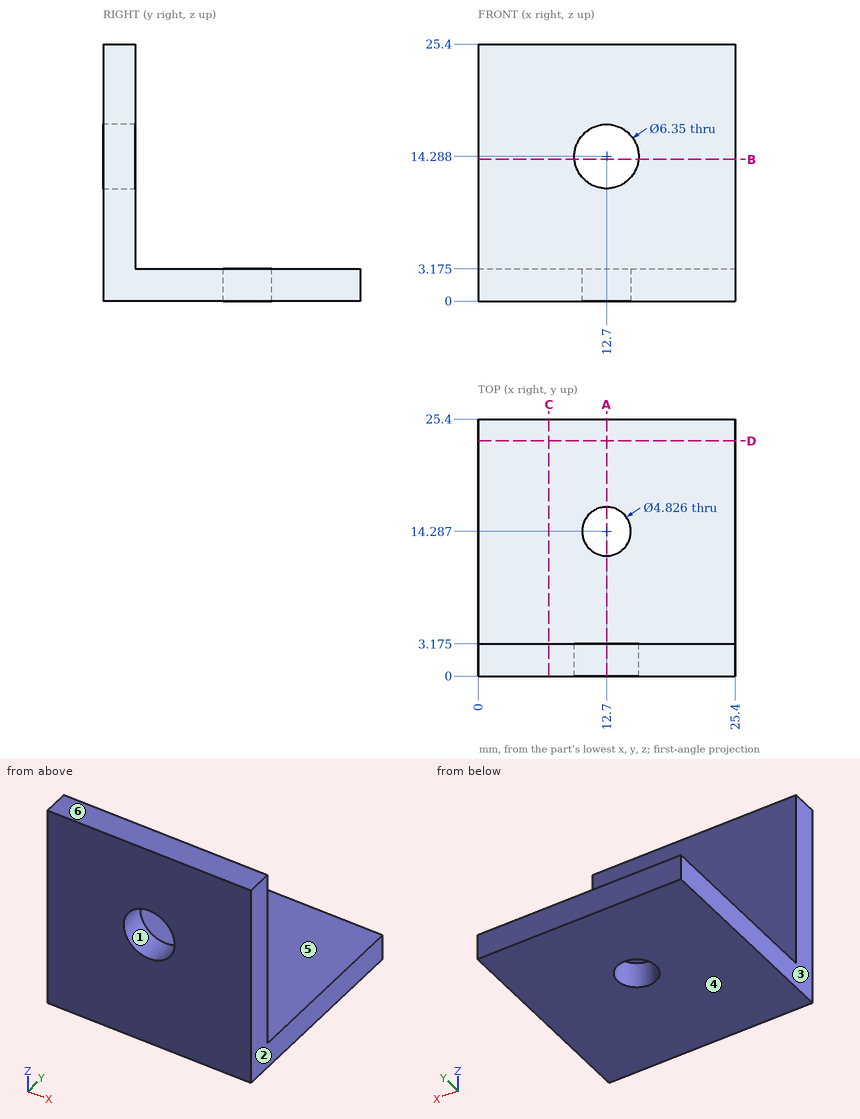
Part print with two shaded views. Sizes in mm from the minimum x, y, z corner. A direction names the side the tool comes from. Round coordinates to 2 decimals unless told otherwise and drop trailing zeros. Write each loop counter-clockwise with the first axis right and the second up, starting at its lowest first coordinate (ties: lowest second). Pieces come first, ordered by that corner, then holes. Notation, with made-up numbers: M 87.25,65.25 L 143.25,65.25 A19 ccw 143.25,72.25 Z; hole C 76.5,15.25 d10. An arc over 180 degrees is marked long. Put each result on its own line as item: value. Start each with the question number.
1) Saw through at B-B, the plane z = 14. Write the cut outline in (x, y) (1 decimal).
2) Saw through at C-C, the plane x = 7. Write the cut outline in (y, z) (1 decimal).
3) Drill centre lines: probe 1 along Y at (x, z) = (12.7, 1.45) (1 decimal); probe 2 along Z at (x, y) = (12, 18.5) (1 decimal). Where is each one in solid material? Low to high. Write a range as [from, to].
4) Saw through at A-A, the plane x = 12.7. Write the cut outline in (y, z) (1 decimal).
5) Saw through at D-D, the plane y = 23.25. Write the cut outline in (x, z) (1 decimal).
6) Pull direction X, two halves, no side cores. Call the marked faces 1, 2, 3 and 4: pulls with the +X half, pulls with the -X half, needs draft (parallel to the pull), parting line crosses it, or undercut.
7) 3-axis set-ups, long thin cutter, end or side, ignore diameter. For the marked faces 5 and 6: which of +Z, -Z, +X, -X, +Y, -Y reach the whole face in a straight line?
8) Pin check, flat tips, straight feed: pin 1 Ø10 at (x, z) = (3, 17.5) entering from +Y (1 decimal); pin 2 Ø6 at (x, y) = (10, 15.5) entering from +Z (1 decimal). Stop position of each tip, or through.
Resolved:
1. outline: M 0,0 L 9.5,0 L 9.5,3.2 L 0,3.2 Z; M 15.9,0 L 25.4,0 L 25.4,3.2 L 15.9,3.2 Z
2. outline: M 0,0 L 25.4,0 L 25.4,3.2 L 3.2,3.2 L 3.2,25.4 L 0,25.4 Z
3. probe 1: [0, 11.9], [16.7, 25.4]
3. probe 2: [0, 3.2]
4. outline: M 0,0 L 11.9,0 L 11.9,3.2 L 3.2,3.2 L 3.2,11.1 L 0,11.1 Z; M 0,17.5 L 3.2,17.5 L 3.2,25.4 L 0,25.4 Z; M 16.7,0 L 25.4,0 L 25.4,3.2 L 16.7,3.2 Z
5. outline: M 0,0 L 25.4,0 L 25.4,3.2 L 0,3.2 Z
6. face 1: undercut
6. face 2: pulls with the +X half
6. face 3: pulls with the -X half
6. face 4: needs draft
7. face 5: +Z, +X, -X, +Y
7. face 6: +Z, +X, -X, +Y, -Y
8. pin 1: y = 3.2
8. pin 2: z = 3.2
